Design review of the part built by this model. Coordinates are the model's own, in mm. Face numbers are marked on the shaded views. Round coordinates to 2 decimals unless told otherwise and drop trailing zeros. Write each loop counter-clockwise with the first axis right and the second up, starting at its lowest first coordinate (ties: lowest second). Pieces come first, ordered by that corner, then holes. Notation, with made-up numbers: M 47,12 L 82,12 A14 ccw 82,31 Z; hole C -6.75,-32 d4. An arc over 180 degrees is marked long. Use CSV: the item, a comma, the result in double quotes.
from build123d import *

# Parameters (mm, degrees)
F0_R     = 75
F1_DEPTH = 5
F2_R     = 19
F3_DEPTH = 5
F3_TAPER = -3
F4_R     = 28.525
F4_R_2   = 26.025
F5_DEPTH = 18
F6_R     = 26.025
F6_R_2   = 24.025
F7_DEPTH = 2


with BuildPart() as f1:
    # F0 (on Front) → F1 (new body)
    with BuildSketch(Plane.XZ):
        Circle(F0_R)
    extrude(amount=F1_DEPTH)

    # F2 (on face) → F3 (cut, through all)
    with BuildSketch(Plane.XZ.offset(5)):
        Circle(F2_R)
    extrude(amount=-F3_DEPTH, taper=F3_TAPER, mode=Mode.SUBTRACT)

    # F4 (on face) → F5 (join)
    with BuildSketch(Plane.XZ.offset(5)):
        Circle(F4_R)
        Circle(F4_R_2, mode=Mode.SUBTRACT)
    extrude(amount=F5_DEPTH)

    # F6 (on face) → F7 (join)
    with BuildSketch(Plane.XZ.offset(5)):
        Circle(F6_R)
        Circle(F6_R_2, mode=Mode.SUBTRACT)
    extrude(amount=F7_DEPTH)


solid = f1.part
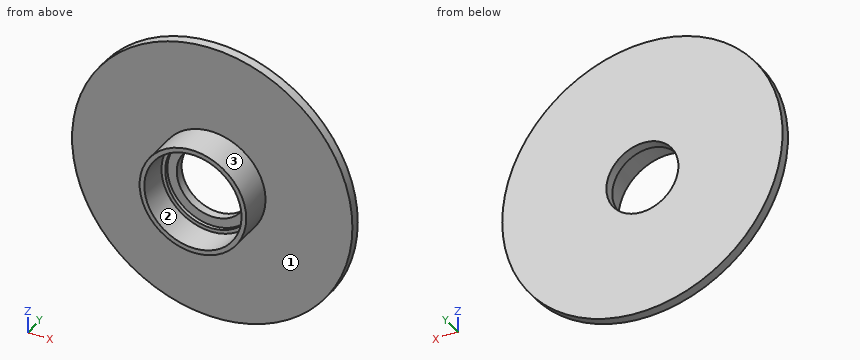
1) Add section D-D on x = -64.5. Write out the cut boundary in (y, z).
Answers:
outline,"M -5,-38.27 L 0,-38.27 L 0,38.27 L -5,38.27 Z"
2) Wall thickness on line 1 along Y through (x, z) = (-54.5, -37.5); line 2 along Z through (x, y) = (0, -6.25) (3 decimals); line 3 along Z through (x, y) = (-23.5, -11.75): over which ranges is each line inside the solid? List them lowest first. Write a range as [from, to].
Answers:
line 1,"[-5, 0]"
line 2,"[-28.525, -24.025], [24.025, 28.525]"
line 3,"[-16.17, -11.18], [11.18, 16.17]"
3) Add section C-C on z = 37. Write out the cut boundary in (x, y), then the cut area to 3 significant figures.
Answers:
outline,"M -65.24,-5 L 65.24,-5 L 65.24,0 L -65.24,0 Z"
area,"652 mm²"
4) The part is to be moulded in two halves that separate along X. For the marked faces 1, 2 and 3, say which applies: released by +X, released by -X, zero draft, split by the parting line, or undercut.
Answers:
face 1,"zero draft"
face 2,"undercut"
face 3,"split by the parting line"
5) For pin 1 Ø3 at (y, z) = (-3.5, -4.5) entering from +X; pin 2 Ø5 at (x, z) = (49, -31.5) entering from +Y; pin 3 Ø1 at (x, y) = (37.5, -7) entering from -Z; pin 4 Ø1 at (y, z) = (-14, -3) entering from +X, all flat-tipped, find the tip position at first contact; note any pin that passes through.
Answers:
pin 1,"x = 74.94"
pin 2,"y = 0"
pin 3,"through"
pin 4,"x = 28.42"
6) Add section A-A on x = 0. Write out the cut boundary in (y, z) (3 decimals).
Answers:
outline,"M -23,-28.525 L -5,-28.525 L -5,-75 L 0,-75 L 0,-19.262 L -5,-19 L -5,-24.025 L -7,-24.025 L -7,-26.025 L -23,-26.025 Z; M -23,26.025 L -7,26.025 L -7,24.025 L -5,24.025 L -5,19 L 0,19.262 L 0,75 L -5,75 L -5,28.525 L -23,28.525 Z"
7) Add section B-B on y = -14. Write out the cut boundary in (x, z) (3 decimals), then the cut area to 3 significant figures.
Answers:
outline,"C 0,0 d57.05; hole C 0,0 d52.05"
area,"428 mm²"
